Verification items for the finished model (mm, model axes). A direction names the side the tool comes from. Round coordinates to 2 decimals unless told otherwise and drop trailing zeros. Write each loop counter-clockwise with the first axis right and the second up, starting at its lowest first coordinate (ties: lowest second). Pieces come first, ordered by that corner, then holes. Notation, with made-up numbers: M -15.75,48.5 L -10.75,48.5 A27 ccw -10.75,71.5 Z; hole C 58.25,-14.5 d5. An arc over 180 degrees is marked long. One line per question, with ' | ' between items.
from build123d import *

# Parameters (mm, degrees)
F1_DEPTH = 63.5
F2_DEPTH = 25.4
F3_DEPTH = 6.35
F0_W     = 50.8
F0_H     = 50.8
F5_R     = 12.7
F6_R     = 14.605
F7_DEPTH = 165.101
F8_R     = 6.35
F9_DEPTH = 63.501


with BuildPart() as f1:
    # F0 (on Front) → F1 (new body, symmetric)
    with BuildSketch(Plane.XZ):
        Polygon((55.88, 31.75), (-63.5, 31.75), (-63.5, -31.75), (63.5, -31.75), (63.5, 31.75), align=None)
    extrude(amount=F1_DEPTH, both=True)

    # F0 (on Front) → F2 (join, symmetric)
    with BuildSketch(Plane.XZ):
        Polygon((139.7, 133.35), (139.7, 110.18212), (139.7, 102.56212), (139.7, 82.55), (190.5, 82.55), (190.5, 133.35), align=None)
        with BuildLine():
            Line((55.88, 64.46212), (55.88, 31.75))
            Line((55.88, 31.75), (63.5, 31.75))
            Line((63.5, 31.75), (63.5, 64.46212))
            ThreePointArc((63.5, 64.46212), (74.659232, 91.402888), (101.6, 102.56212))
            Line((101.6, 102.56212), (139.7, 102.56212))
            Line((139.7, 102.56212), (139.7, 110.18212))
            Line((139.7, 110.18212), (101.6, 110.18212))
            ThreePointArc((101.6, 110.18212), (69.271078, 96.791042), (55.88, 64.46212))
        make_face()
    extrude(amount=F2_DEPTH, both=True)

    # F0 (on Front) → F3 (join, symmetric)
    with BuildSketch(Plane.XZ):
        with BuildLine():
            add(Edge.make_bspline(
                [(-63.5, 31.75), (-41.28221, 95.252596), (30.595858, 110.611163), (101.6, 110.18212)],
                knots=[0, 0, 0, 0, 182.782952, 182.782952, 182.782952, 182.782952], degree=3))
            Line((-63.5, 31.75), (55.88, 31.75))
            Line((55.88, 31.75), (55.88, 64.46212))
            ThreePointArc((55.88, 64.46212), (69.271078, 96.791042), (101.6, 110.18212))
        make_face()
    extrude(amount=F3_DEPTH, both=True)

    # F0 (on Front) → F4 (revolve)
    with BuildSketch(Plane.XZ):
        with Locations((215.9, 107.95)):
            Rectangle(F0_W, F0_H)
    revolve(axis=Axis((190.5, 0, 107.95), (0, 0, 1)))

    # F5
    f5_edges = [f1.edges().sort_by_distance(p)[0] for p in [
        (63.5, -63.5, 0),
        (-63.5, -63.5, 0),
        (-63.5, 63.5, 0),
        (63.5, 63.5, 0),
    ]]
    fillet(f5_edges, radius=F5_R)

    # F6 (on face) → F7 (cut, through all)
    with BuildSketch(Plane.XY.offset(133.35)):
        with Locations((190.5, 0)):
            Circle(F6_R)
    extrude(amount=-F7_DEPTH, mode=Mode.SUBTRACT)

    # F8 (on face) → F9 (cut, through all)
    with BuildSketch(Plane.XY.offset(31.75)):
        with Locations((-38.1, -38.1)):
            Circle(F8_R)
        with Locations((38.1, -38.1)):
            Circle(F8_R)
        with Locations((38.1, 38.1)):
            Circle(F8_R)
        with Locations((-38.1, 38.1)):
            Circle(F8_R)
    extrude(amount=-F9_DEPTH, mode=Mode.SUBTRACT)


solid = f1.part
1. Mould release check, pull along Y, two halves, no side actions. Record for faces 6 (the face through (63.5, -1, 5)), 7 (the face through (-35.17, 32.466, 0.444)), 8 (the face through (59.68, 59.88, 0.44)): pulls with the +Y half, pulls with the -Y half, needs draft (parallel to the pull), parting line crosses it, or undercut.
Results:
face 6: needs draft | face 7: undercut | face 8: pulls with the +Y half
2. Section check B-B, the plane z = 8. Record the cut outline in (x, y).
Results:
outline: M -63.5,-50.8 A12.7 ccw -50.8,-63.5 L 50.8,-63.5 A12.7 ccw 63.5,-50.8 L 63.5,50.8 A12.7 ccw 50.8,63.5 L -50.8,63.5 A12.7 ccw -63.5,50.8 Z; hole C -38.1,-38.1 d12.7; hole C -38.1,38.1 d12.7; hole C 38.1,-38.1 d12.7; hole C 38.1,38.1 d12.7
3. Go/stop test with flat-tipped pins: P1, Ø15, axis at y = -17.5, z = 48.5, coming from the -X side; P2, Ø1, axis at x = 65, y = 45, coming from the -Z side; P3, Ø8, axis at x = 155.5, y = -10, coming from the -Z side; P4, Ø23.5, axis at x = 33.5, z = 60.5, coming from the -Y side. Record where each tip stops, or that it passes through.
Results:
P1: stops at x = 55.88 | P2: passes through | P3: stops at z = 82.55 | P4: stops at y = -6.35
4. Tool access check on faces 1 (the face through (139.7, 0, 122)), 2 (the face through (-59.88, -59.68, -0.44)), 3 (the face through (2, 6.35, 63)), 4 (the face through (1, -35, 31.75)), 5 (the face through (180, -11, 82.55)). Record the directions out of +Z, -Z, +X, -X, +Y, -Y that give a thin tool (end or side, any length) a straight path to the whole face; none if there is none.
Results:
face 1: +Z, -X, +Y, -Y | face 2: +Z, -Z, -X, -Y | face 3: +Z, -X, +Y | face 4: +Z, -X, -Y | face 5: -Z, +X, +Y, -Y
5. Section check D-D, the plane z = 122. Record the cut outline in (x, y) (3 decimals).
Results:
outline: M 139.7,-25.4 L 146.506,-25.4 A50.8 ccw long 146.506,25.4 L 139.7,25.4 Z; hole C 190.5,0 d29.21
6. Section check C-C, the plane y = 38.1. Record the cut outline in (x, z).
Results:
outline: M -63.5,-31.75 L -44.45,-31.75 L -44.45,31.75 L -63.5,31.75 Z; M -31.75,-31.75 L 31.75,-31.75 L 31.75,31.75 L -31.75,31.75 Z; M 44.45,-31.75 L 63.5,-31.75 L 63.5,31.75 L 44.45,31.75 Z; M 156.9,82.55 L 224.1,82.55 L 224.1,133.35 L 156.9,133.35 Z
7. Thickness scan on line 1 (X direction, y = -38, z = -2); line 2 (Y direction, x = 190.5, z = 106) (3 decimals). Record the ranges inside material, lowest first.
Results:
line 1: x = -63.5 to -44.45, -31.75 to 31.75, 44.45 to 63.5 | line 2: y = -50.8 to -14.605, 14.605 to 50.8
8. Section check A-A, the plane x = 190.5. Record the cut outline in (y, z) (3 decimals), then the cut area to 3 significant figures.
Results:
outline: M -50.8,82.55 L -14.605,82.55 L -14.605,133.35 L -50.8,133.35 Z; M 14.605,82.55 L 50.8,82.55 L 50.8,133.35 L 14.605,133.35 Z | area: 3,680 mm2
